```python
from build123d import *

# Parameters (mm, degrees)
F0_W      = 20
F0_H      = 25
F1_DEPTH  = 80
F2_R      = 5
F2_R_2    = 4.5
F3_DEPTH  = 25
F5_DEPTH  = 52.5
F6_W      = 25
F6_H      = 80
F7_DEPTH  = 30
F9_DEPTH  = 20
F10_R     = 12.5
F11_DEPTH = 30


with BuildPart() as f1:
    # F0 (on Top) → F1 (new body)
    with BuildSketch(Plane.XY):
        with Locations((10, -12.5)):
            Rectangle(F0_W, F0_H)
    extrude(amount=F1_DEPTH)

    # F2 (on face) → F3 (cut)
    with BuildSketch(Plane.YZ.offset(20)):
        with Locations((-12.5, 71)):
            Circle(F2_R)
        with Locations((-12.5, 56)):
            Circle(F2_R_2)
        with Locations((-12.5, 41)):
            Circle(F2_R)
        with Locations((-12.5, 26)):
            Circle(F2_R_2)
    extrude(amount=-F3_DEPTH, mode=Mode.SUBTRACT)

    # F4 (on face) → F5 (join)
    with BuildSketch(Plane.XZ.offset(25)):
        Polygon((-25, 0), (0, 0), (50, 0), (50, 80), (-25, 80), align=None)
    extrude(amount=F5_DEPTH)

    # F6 (on face) → F7 (join)
    with BuildSketch(Plane.YZ.offset(20)):
        with Locations((-12.5, 40)):
            Rectangle(F6_W, F6_H)
    extrude(amount=F7_DEPTH)

    # F8 (on face) → F9 (join)
    with BuildSketch(Plane(origin=(0, 0, 0), x_dir=(1, 0, 0), z_dir=(0, 0, -1))):
        Polygon((-25, 77.5), (-25, 25), (0, 25), (0, 0), (50, 0), (50, 77.5), align=None)
    extrude(amount=F9_DEPTH)

    # F10 (on face) → F11 (join)
    with BuildSketch(Plane(origin=(0, 0, 0), x_dir=(-1, 0, 0), z_dir=(0, 1, 0))):
        with Locations((-25, 10)):
            Circle(F10_R)
    extrude(amount=F11_DEPTH)


solid = f1.part
```
Here's how the part is built. I have some questions about the finished solid (model axes, mm). A direction names the side the tool comes from. Coordinates: 2 decimals unless noted, no trailing zeros. Order: outer loops, then holes, each group sorted by start corner. A loop starts at its lowest first (then second) coordinate and runs counter-clockwise, first axis right, second up.
1) Imagine slicing it at D-D on z = 71. List the corners of the cut face in (x, y) for me, and give its area (3 significant figures).
2) Will these pins go through, and if not, where does the flat tip stop? pin 1 (12 mm diameter, centred on x = -5.5, y = -1.5, fed in from -Z); pin 2 (10 mm diameter, centred on y = -11.5, z = 25, fed in from -X); pin 3 (3 mm diameter, centred on y = -12.5, z = 39.5, fed in from -X); pin 4 (10 mm diameter, centred on y = 6.5, z = 19, fed in from -X).
3) I need wall thicknesses on line 1 (Z direction, x = 10.5, y = -12.5); line 2 (Y direction, x = -10, z = -2); line 3 (X direction, y = -22.5, z = 2.5). Which ranges of each line are inside material? Lowest first, please.
4) Imagine slicing it at C-C on y = -12.5. List the corners of the cut face in (x, z) for me.
5) Which directions (+Z, -Z, +X, -X, +Y, -Y) give clear straight access to the entire face, cutting with the end or side of a thin tool? Please do faces 5 (the face through (34.92, 14.79, 2.394)), 6 (the face through (0, -13, 31)), 7 (the face through (10.14, -10.081, 29.794)), 8 (the face through (-25, -52, 31)).
6) Imagine slicing it at B-B on z = 10. List the corners of the cut face in (x, y) for me.
7) Imagine slicing it at A-A on x = 15. List the corners of the cut face in (y, z) for me.
8) We'd pull the mould along Y, two halves only. Please class faces 1 (the face through (20, -13, 26)), 2 (the face through (12, -39, 80)), 3 (the face through (-13, -25, 31)), 4 (the face through (10.14, -10.42, 52.01)): +Y half, -Y half, draft (parallel to the pull), parting line (faces both ways), or undercut.
Response values:
1. outline: (-25, -77.5) - (50, -77.5) - (50, 0) - (0, 0) - (0, -7.5) - (20, -7.5) - (20, -17.5) - (0, -17.5) - (0, -25) - (-25, -25) - close
1. area: 4,990 mm2
2. pin 1: stops at z = -20
2. pin 2: stops at x = 0
2. pin 3: stops at x = 20
2. pin 4: stops at x = 13.16
3. line 1: z = -20 to 21.5, 30.5 to 36, 46 to 51.5, 60.5 to 66, 76 to 80
3. line 2: y = -77.5 to -25
3. line 3: x = 0 to 50
4. outline: (0, -20) - (50, -20) - (50, 80) - (0, 80) - (0, 76) - (20, 76) - (20, 66) - (0, 66) - (0, 60.5) - (20, 60.5) - (20, 51.5) - (0, 51.5) - (0, 46) - (20, 46) - (20, 36) - (0, 36) - (0, 30.5) - (20, 30.5) - (20, 21.5) - (0, 21.5) - close
5. face 5: +Y
5. face 6: +Z, -Z, -X, +Y
5. face 7: -X
5. face 8: +Z, -Z, -X, +Y, -Y
6. outline: (-25, -77.5) - (50, -77.5) - (50, 0) - (37.5, 0) - (37.5, 30) - (12.5, 30) - (12.5, 0) - (0, 0) - (0, -25) - (-25, -25) - close
7. outline: (-77.5, -20) - (0, -20) - (0, 2.5) - (30, 2.5) - (30, 17.5) - (0, 17.5) - (0, 80) - (-77.5, 80) - close; hole circle Ø10 at (-12.5, 41); hole circle Ø10 at (-12.5, 71); hole circle Ø9 at (-12.5, 26); hole circle Ø9 at (-12.5, 56)
8. face 1: undercut
8. face 2: draft
8. face 3: +Y half
8. face 4: undercut
